Design review of the part built by this model. Coordinates are the model's own, in mm. Face numbers are marked on the shaded views. Coordinates: 2 decimals unless noted, no trailing zeros. Loops run counter-clockwise (first coordinate to the right, second up) from the corner with the lowest first, then second, coordinate; pieces in that order, holes last. Notation, with made-up numbers: M -37,-27 L 20,-27 A21 cw 20,11 Z; hole C -16.5,-28.5 d2. An arc over 180 degrees is marked long. Answer as CSV lines item,"result". Start each with the question number.
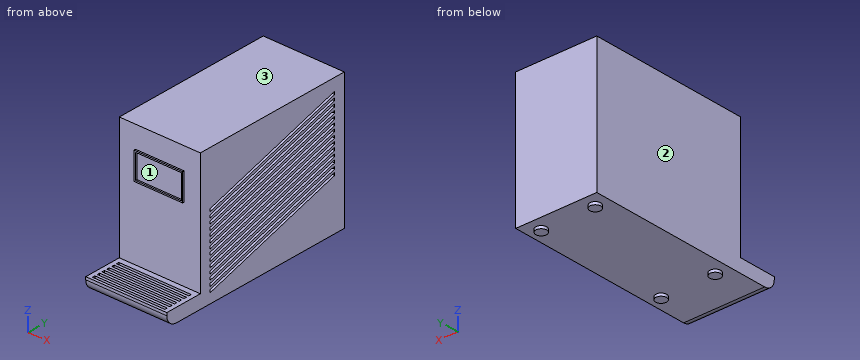
from build123d import *

# Parameters (mm, degrees)
F0_W      = 38.1
F0_H      = 76.2
F1_DEPTH  = 63.5
F3_R      = 2.54
F4_DEPTH  = 1.27
F6_DEPTH  = 25.4
F8_DEPTH  = 38.1
F9_W      = 38.1
F9_H      = 17.78
F10_DEPTH = 1.27
F11_W     = 34.036
F11_H     = 1.27
F12_DEPTH = 2.54
F2_W      = 22.86
F2_H      = 12.7
F2_W_2    = 21.59
F2_H_2    = 11.43
F13_DEPTH = 0.762


with BuildPart() as f1:
    # F0 (on Top) → F1 (new body)
    with BuildSketch(Plane.XY):
        Rectangle(F0_W, F0_H)
    extrude(amount=F1_DEPTH)

    # F3 (on face) → F4 (join)
    with BuildSketch(Plane(origin=(0, 0, 0), x_dir=(1, 0, 0), z_dir=(0, 0, -1))):
        with Locations((-12.7, 31.75)):
            Circle(F3_R)
        with Locations((12.7, 31.75)):
            Circle(F3_R)
        with Locations((-12.7, -31.75)):
            Circle(F3_R)
        with Locations((12.7, -31.75)):
            Circle(F3_R)
    extrude(amount=F4_DEPTH)

    # F5 (on face) → F6 (cut)
    with BuildSketch(Plane.YZ.offset(19.05)):
        Polygon((33.02, 57.846099), (-33.02, 38.635515), (-33.02, 37.365515), (33.02, 56.576099), align=None)
        Polygon((-33.02, 25.990401), (-33.02, 24.720401), (33.02, 43.930985), (33.02, 45.200985), align=None)
        Polygon((-33.02, 28.530401), (-33.02, 27.260401), (33.02, 46.470985), (33.02, 47.740985), align=None)
        Polygon((-33.02, 31.042958), (-33.02, 29.772958), (33.02, 48.983542), (33.02, 50.253542), align=None)
        Polygon((-33.02, 33.582958), (-33.02, 32.312958), (33.02, 51.523542), (33.02, 52.793542), align=None)
        Polygon((-33.02, 36.095515), (-33.02, 34.825515), (33.02, 54.036099), (33.02, 55.306099), align=None)
        Polygon((33.02, 42.688428), (-33.02, 23.477843), (-33.02, 22.207843), (33.02, 41.418428), align=None)
        Polygon((-33.02, 20.937843), (-33.02, 19.667843), (33.02, 38.878428), (33.02, 40.148428), align=None)
        Polygon((-33.02, 15.885286), (-33.02, 14.615286), (33.02, 33.825871), (33.02, 35.095871), align=None)
        Polygon((-33.02, 18.425286), (-33.02, 17.155286), (33.02, 36.365871), (33.02, 37.635871), align=None)
        Polygon((-33.02, 10.832729), (-33.02, 9.562729), (33.02, 28.773313), (33.02, 30.043313), align=None)
        Polygon((-33.02, 13.372729), (-33.02, 12.102729), (33.02, 31.313313), (33.02, 32.583313), align=None)
        Polygon((-33.02, 5.780172), (-33.02, 4.510172), (33.02, 23.720756), (33.02, 24.990756), align=None)
        Polygon((-33.02, 8.320172), (-33.02, 7.050172), (33.02, 26.260756), (33.02, 27.530756), align=None)
    extrude(amount=-F6_DEPTH, mode=Mode.SUBTRACT)

    # F7 (on face) → F8 (join)
    with BuildSketch(Plane(origin=(-19.05, 0, 0), x_dir=(0, -1, 0), z_dir=(-1, 0, 0))):
        with BuildLine():
            Line((38.1, 5.08), (38.1, 0))
            Line((38.1, 0), (50.8, 0))
            ThreePointArc((50.8, 0), (54.392102, 1.487898), (55.88, 5.08))
            Line((55.88, 5.08), (50.8, 5.08))
            Line((50.8, 5.08), (38.1, 5.08))
        make_face()
    extrude(amount=-F8_DEPTH)

    # F9 (on face) → F10 (join)
    with BuildSketch(Plane.XY.offset(5.08)):
        with Locations((0, -46.99)):
            Rectangle(F9_W, F9_H)
    extrude(amount=F10_DEPTH)

    # F11 (on face) → F12 (cut)
    with BuildSketch(Plane.XY.offset(6.35)):
        with Locations((0, -41.275)):
            Rectangle(F11_W, F11_H)
        Polygon((17.018, -43.269459), (17.018, -43.18), (-17.018, -43.18), (-17.018, -44.45), (17.018, -44.45), align=None)
        with Locations((0, -46.355)):
            Rectangle(F11_W, F11_H)
        with Locations((0, -48.895)):
            Rectangle(F11_W, F11_H)
        with Locations((0, -51.435)):
            Rectangle(F11_W, F11_H)
        with Locations((0, -53.975)):
            Rectangle(F11_W, F11_H)
    extrude(amount=-F12_DEPTH, mode=Mode.SUBTRACT)

    # F2 (on face) → F13 (join)
    with BuildSketch(Plane.XZ.offset(38.1)):
        with Locations((0, 46.947837)):
            Rectangle(F2_W, F2_H)
        with Locations((0, 46.947837)):
            Rectangle(F2_W_2, F2_H_2, mode=Mode.SUBTRACT)
    extrude(amount=F13_DEPTH)


solid = f1.part
Item 1: Add section A-A (x = 12.7). Give the number of separate pieces and of enclosed holes in the cut face, plus the area to 3 significant figures.
Item 2: For pin 1 (0.6 mm diameter, centred on y = -38.5, z = 44.5, fed in from +X); pin 2 (0.6 mm diameter, centred on x = 6, z = 31.5, fed in from -Y); pin 3 (1 mm diameter, centred on x = -3, y = -43.5, fed in from +Z); pin 4 (16.5 mm diameter, centred on y = 7.5, z = 26.5, fed in from +X), all flat-tipped, find the tip position at first contact; note any pin that passes through.
Item 3: For line 1 along Y through (x, z) = (-11, 38); line 2 along Z through (x, y) = (-5.5, -51); line 3 along Z through (x, y) = (-11, -7.5), list the stretches that pass through material, from the lowest coordinate up. Write a range as from..to.
Item 4: Add section B-B (z = 59). Give the boundary of the cut face in (x, y).
Item 5: Mouldability with a two-part tool opening along X and no side actions: class the marked faces 1, 2 and 3 as released by +X, released by -X, zero draft, split by the parting line, or undercut.
Response:
1,separate pieces,"1"
1,enclosed holes,"14"
1,area,"3,770 mm²"
2,pin 1,"x = 11.43"
2,pin 2,"y = -38.1"
2,pin 3,"z = 6.35"
2,pin 4,"x = 19.05"
3,line 1,"-38.1..38.1"
3,line 2,"0..3.81"
3,line 3,"0..63.5"
4,outline,"M -19.05,-38.1 L 19.05,-38.1 L 19.05,38.1 L -19.05,38.1 Z"
5,face 1,"undercut"
5,face 2,"released by -X"
5,face 3,"zero draft"
